Work out the finished part from the listing and answer in its coordinate system (mm). A direction names the side the tool comes from. Give positions to 0.01 mm unless a question says otherwise; leave off trailing zeros. Write each loop counter-clockwise with the first axis right and the second up, starting at its lowest first coordinate (ties: lowest second). Pieces come first, ordered by that corner, then holes. Notation, with made-up numbers: (63.5, -4.5) -> (114.5, -4.5) arc R36 ccw to (114.5, 34.5) -> close; hole circle Ø4 at (-7.5, 41.25). An arc over 180 degrees is marked (long way). Use a Markdown table: item, result. Add a question column.
Q1. Consider line 1 (Y direction, x = -3, z = -8.25); line 2 (X direction, y = -141.5, z = 0.25); line 3 (Y direction, x = 174, z = -0.5). Determine where each line is inside the solid, lowest interval first.
Q2. For a pull along X with two mould halves and no side action, classify faces 5 (the face through (0, -250, 0)), 6 (the face through (-11.923, 7.888, 3.755)), 7 (the face through (215, 54, 0)) as pulls with the +X half, pulls with the -X half, needs draft (parallel to the pull), parting line crosses it, or undercut.
Q3. Each of these flat-tipped pins is pushed along its axis until it touches: pin 1 Ø4 at (x, z) = (168.5, 6.5) entering from +Y; pin 2 Ø10 at (x, z) = (95, -2) entering from +Y; pin 3 Ø6 at (x, z) = (71.5, 0.5) entering from +Y. Where does it stop, or does it pass through?
Q4. Section A-A, the plane y = -35.5 is taken. Give the vertices of the cut face in (x, z), plus the area to 3 significant figures.
Q5. For faces 1 (the face through (-11.923, -241.888, 3.755)), 2 (the face through (215, -288, 0)), 3 (the face through (0.2, 0, -8.2)), 4 (the face through (0, 16, 0)), determine the directions among +Z, -Z, +X, -X, +Y, -Y from which every point of the face is accessible in a straight line to the end or side of a thin tool.
Q6. Section B-B, the plane z = 0 is taken. Give the vertices of the cut face in (x, y), plus the area to 3 significant figures.
from build123d import *

# Parameters (mm, degrees)
F0_R     = 8
F1_DEPTH = 234
F2_R     = 12.5
F2_R_2   = 8
F3_DEPTH = 16
F4_R     = 12.5
F5_DEPTH = 16
F7_W     = 95.3162200749
F7_H     = 152.7085006237
F8_DEPTH = 50
F10_R    = 8


with BuildPart() as f1:
    # F0 (on Front) → F1 (new body)
    with BuildSketch(Plane.XZ):
        Circle(F0_R)
    extrude(amount=F1_DEPTH)

    # F2 (on face) → F3 (join)
    with BuildSketch(Plane.XZ.offset(234)):
        Circle(F2_R)
        Circle(F2_R_2, mode=Mode.SUBTRACT)
        Circle(F2_R_2)
    extrude(amount=F3_DEPTH)

    # F4 (on face) → F5 (join)
    with BuildSketch(Plane(origin=(0, 0, 0), x_dir=(-1, 0, 0), z_dir=(0, 1, 0))):
        Circle(F4_R)
    extrude(amount=F5_DEPTH)

    # F7 (on Top) → F8 (cut, symmetric)
    with BuildSketch(Plane.XY):
        with Locations((7.3376540095, -193.3542503119)):
            Rectangle(F7_W, F7_H)
    extrude(amount=F8_DEPTH, both=True, mode=Mode.SUBTRACT)

    # F11: sweep along a path in F6
    with BuildLine(Plane.XY) as f11_path:
        Line((0, -22), (215, 54))
    # F10 (on line) → F11 (sweep)
    with BuildSketch(Plane(origin=(-6.9129439818, -2.4436453145, 0), x_dir=(-0.3332788427, 0.9428283051, 0), z_dir=(0.9428283051, 0.3332788427, 0))):
        with Locations((-20.7422227131, 0)):
            Circle(F10_R)
    sweep(path=f11_path.line)

    # F12: F1 across face


with BuildPart() as f1_1:
    add(f1.part)
    add(f1.part.mirror(Plane.XZ.offset(117)))


solid = f1_1.part
Result set:
| question | item | result |
|---|---|---|
| 1 | line 1 | y = -250 to -234, 0 to 16 |
| 1 | line 2 | x = -8 to 8 |
| 1 | line 3 | y = -281.98 to -265.04, 31.04 to 47.98 |
| 2 | face 5 | needs draft |
| 2 | face 6 | undercut |
| 2 | face 7 | pulls with the +X half |
| 3 | pin 1 | stops at y = 44.74 |
| 3 | pin 2 | stops at y = 21.74 |
| 3 | pin 3 | stops at y = 12.81 |
| 4 | outline | circle Ø16 at (0, 0) |
| 4 | area | 201 mm2 |
| 5 | face 1 | -Y |
| 5 | face 2 | +Z, -Z, +X, -Y |
| 5 | face 3 | none |
| 5 | face 4 | +Z, -Z, -X, +Y |
| 6 | outline | (-12.5, -250) -> (12.5, -250) -> (12.5, -234) -> (8, -234) -> (8, -223.31) -> (212.33, -295.54) -> (217.67, -280.46) -> (8, -206.34) -> (8, -27.66) -> (217.67, 46.46) -> (212.33, 61.54) -> (8, -10.69) -> (8, 0) -> (12.5, 0) -> (12.5, 16) -> (-12.5, 16) -> (-12.5, 0) -> (-8, 0) -> (-8, -234) -> (-12.5, -234) -> close |
| 6 | area | 11,600 mm2 |
